```python
from build123d import *

# Parameters (mm, degrees)
F0_W      = 101
F0_H      = 2
F1_DEPTH  = 12
F0_H_2    = 71
F2_DEPTH  = 2
F4_R      = 1.75
F5_DEPTH  = 100
F3_W      = 49
F3_H      = 12
F6_DEPTH  = 2
F7_W      = 35
F7_H      = 50
F7_W_2    = 30
F8_DEPTH  = 2
F9_W      = 5.5
F9_H      = 2
F10_DEPTH = 80


with BuildPart() as f1:
    # F0 (on Top) → F1 (new body)
    with BuildSketch(Plane.XY):
        Polygon((-42.37669, -41.099664), (-42.37669, 29.900336), (-42.37669, 31.900336), (-44.37669, 31.900336), (-44.37669, -43.099664), (-42.37669, -43.099664), align=None)
        with Locations((8.12331, 30.900336)):
            Rectangle(F0_W, F0_H)
        Polygon((58.62331, 31.900336), (58.62331, 29.900336), (58.62331, -41.099664), (58.62331, -43.099664), (60.62331, -43.099664), (60.62331, 31.900336), align=None)
        with Locations((8.12331, -42.099664)):
            Rectangle(F0_W, F0_H)
    extrude(amount=F1_DEPTH)

    # F0 (on Top) → F2 (join)
    with BuildSketch(Plane.XY):
        with Locations((8.12331, -5.599664)):
            Rectangle(F0_W, F0_H_2)
    extrude(amount=F2_DEPTH)

    # F4 (on face) → F5 (cut)
    with BuildSketch(Plane.XZ.offset(43.099664)):
        with Locations((44.623323, 5.000008)):
            Circle(F4_R)
        with Locations((-32.376677, 5.000008)):
            Circle(F4_R)
    extrude(amount=-F5_DEPTH, mode=Mode.SUBTRACT)

    # F3 (on face) → F6 (cut)
    with BuildSketch(Plane.YZ.offset(60.62331)):
        with Locations((-10.59967, 6)):
            Rectangle(F3_W, F3_H)
    extrude(amount=-F6_DEPTH, mode=Mode.SUBTRACT)

    # F7 (on face) → F8 (cut)
    with BuildSketch(Plane.XY.offset(2)):
        with Locations((-14.876692, -6.099655)):
            Rectangle(F7_W, F7_H)
        with Locations((32.623308, -6.099655)):
            Rectangle(F7_W_2, F7_H)
    extrude(amount=-F8_DEPTH, mode=Mode.SUBTRACT)

    # F9 (on face) → F10 (cut)
    with BuildSketch(Plane.XZ.offset(43.099664)):
        with Locations((-34.626723, 11.000004)):
            Rectangle(F9_W, F9_H)
        with Locations((6.373277, 11.000004)):
            Rectangle(F9_W, F9_H)
        with Locations((47.373277, 11.000004)):
            Rectangle(F9_W, F9_H)
    extrude(amount=-F10_DEPTH, mode=Mode.SUBTRACT)


solid = f1.part
```
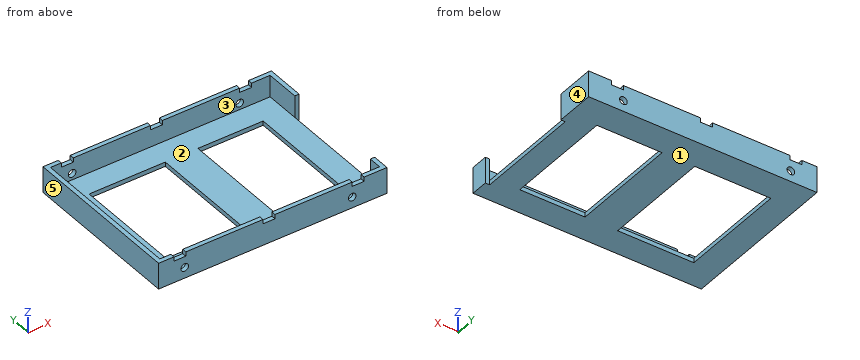
The listing builds one solid part. Answer for the finished solid, in the listing's coordinates (mm). Face numbers are marked on the shaded views. A direction names the side the tool comes from. Give positions to 0.01 mm unless a question says otherwise; leave off trailing zeros. Order: outer loops, then holes, each group sorted by start corner. A loop starts at its lowest first (then second) coordinate and runs counter-clockwise, first axis right, second up. Notation, with made-up numbers: (-18.75, -35.5) -> (3.25, -35.5) arc R31 cw to (3.25, 0.5) -> close; hole circle Ø5 at (14.5, 28). An arc over 180 degrees is marked (long way). One line per item, written item: value.
1) Find the intervals of material crossed by line 1 (Y direction, x = 38.5, z = 11); line 2 (X direction, y = 9.5, z = 0.5); line 3 (X direction, y = 22, z = 3.25), in increasing order.
Reported:
line 1: y = -43.1 to -41.1, 29.9 to 31.9
line 2: x = -44.38 to -32.38, 2.62 to 17.62, 47.62 to 58.62
line 3: x = -44.38 to -42.38, 58.62 to 60.62
2) Find section A-A, the plane y = 9. Determine the outline of the cut face in (x, z), plus the area to 3 significant figures.
Reported:
outline: (-44.38, 0) -> (-32.38, 0) -> (-32.38, 2) -> (-42.38, 2) -> (-42.38, 12) -> (-44.38, 12) -> close; (2.62, 0) -> (17.62, 0) -> (17.62, 2) -> (2.62, 2) -> close; (47.62, 0) -> (58.62, 0) -> (58.62, 2) -> (47.62, 2) -> close
area: 96.0 mm^2
3) Determine the mould class of the marked faces 3, 4 and 5 for opening direction X: pulls with the +X half, pulls with the -X half, needs draft (parallel to the pull), parting line crosses it, or undercut.
Reported:
face 3: undercut
face 4: pulls with the +X half
face 5: pulls with the -X half
4) Find section D-D, the plane y = 25. Determine the outline of the cut face in (x, z), plus the area to 3 significant figures.
Reported:
outline: (-44.38, 0) -> (60.62, 0) -> (60.62, 12) -> (58.62, 12) -> (58.62, 2) -> (-42.38, 2) -> (-42.38, 12) -> (-44.38, 12) -> close
area: 250 mm^2
5) Find section B-B, the plane x = 24.5. Determine the outline of the cut face in (y, z), plus the area to 3 significant figures.
Reported:
outline: (-43.1, 0) -> (-31.1, 0) -> (-31.1, 2) -> (-41.1, 2) -> (-41.1, 12) -> (-43.1, 12) -> close; (18.9, 0) -> (31.9, 0) -> (31.9, 12) -> (29.9, 12) -> (29.9, 2) -> (18.9, 2) -> close
area: 90.0 mm^2
6) Flat-ended cylindrical pins translate along their axes: P1, Ø1, axis at x = 6, y = -42, coming from the +Z side; P2, Ø2, axis at y = 4, z = 2.5, coming from the +X side; P3, Ø6, axis at x = 19, y = -14.5, coming from the +Z side; P4, Ø3, axis at x = -8, y = 22.5, coming from the -Z side. Find the tip coordinate at first contact, or state that the pin passes through.
Reported:
P1: stops at z = 10
P2: stops at x = 58.62
P3: stops at z = 2
P4: stops at z = 0
7) Find section C-C, the plane z = 8.5. Determine the outline of the cut face in (x, y).
Reported:
outline: (-44.38, -43.1) -> (60.62, -43.1) -> (60.62, -35.1) -> (58.62, -35.1) -> (58.62, -41.1) -> (-42.38, -41.1) -> (-42.38, 29.9) -> (58.62, 29.9) -> (58.62, 13.9) -> (60.62, 13.9) -> (60.62, 31.9) -> (-44.38, 31.9) -> close
8) A tool of negligible diameter and unlimited length cuts with its end or side. For the marked faces 1 and 2, from which of +Z, -Z, +X, -X, +Y, -Y can it reach the whole face along a straight path? Write none if from no direction.
Reported:
face 1: -Z, +X, -X, +Y, -Y
face 2: +Z
